Could you check a few things on this model? Use its own coordinates, in mm. Face numbers are marked on the shaded views. Round coordinates to 2 decimals unless told otherwise and drop trailing zeros. Write each question's results on one line, items separated by ' | '. Start each with the question number.
1) If I drill on probe 1 along X at (y, z) = (-11.8, 6.5); probe 2 along Z at (x, y) = (41.25, -11.3); probe 3 along Z at (x, y) = (42.75, -13.25), over which ranges is the centre line in solid material (lowest first)?
2) For P1, Ø3, axis at x = 44.5, z = 8, coming from the +Y side; P2, Ø1.5, axis at x = 44.5, z = 6, coming from the +Y side; P3, Ø1, axis at y = -11.5, z = 5.5, coming from the -X side, each with a flat end and sliding along its axis, tell me the tip position at first contact or that it passes through.
3) We'd pull the mould along Z, two halves only. Please class the marked faces 1 and 2: pulls with the +Z half, pulls with the -Z half, needs draft (parallel to the pull), parting line crosses it, or undercut.
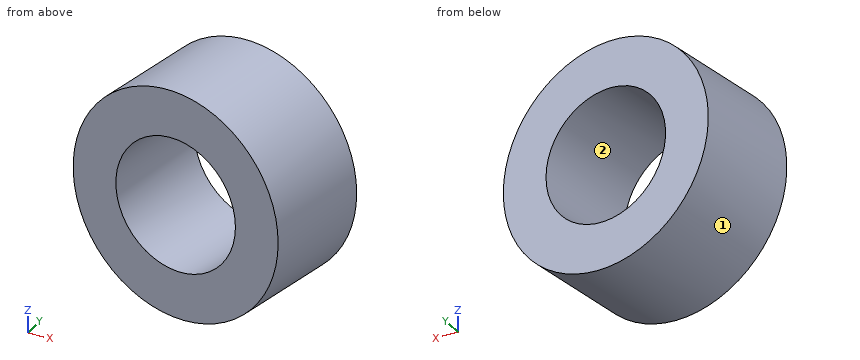
from build123d import *

# Parameters (mm, degrees)
CYLINDER044_R               = 1.75
CYLINDER044_DEPTH           = 18
CYLINDER044_ROLL_ANGLE      = -89.999776
CYLINDER044_PITCH_ANGLE     = 1.4e-05
CYLINDER044_PLACEMENT_ANGLE = -9.999925
CYLINDER045_R               = 3
CYLINDER045_DEPTH           = 3
CYLINDER045_ROLL_ANGLE      = -89.999776
CYLINDER045_PITCH_ANGLE     = 1.4e-05
CYLINDER045_PLACEMENT_ANGLE = -9.999925


with BuildPart() as cylinder044:
    # Cylinder044 → Cylinder044 (new body)
    with BuildSketch(Plane.XY):
        Circle(CYLINDER044_R)
    extrude(amount=CYLINDER044_DEPTH)


with BuildPart() as cylinder044_1:
    # Cylinder044 roll: moved
    add(cylinder044.part.rotate(Axis((0, 0, 0), (1, 0, 0)), CYLINDER044_ROLL_ANGLE))


with BuildPart() as cylinder044_2:
    # Cylinder044 pitch: moved
    add(cylinder044_1.part.rotate(Axis((0, 0, 0), (0, 1, 0)), CYLINDER044_PITCH_ANGLE))


with BuildPart() as cylinder044_3:
    # Cylinder044 placement: moved
    add(cylinder044_2.part.moved(Location((39.936529, -25.15494, 7.500007))).rotate(Axis((39.936529, -25.15494, 7.500007), (0, 0, 1)), CYLINDER044_PLACEMENT_ANGLE))


with BuildPart() as cut037:
    # Cylinder045 → Cylinder045 (new body)
    with BuildSketch(Plane.XY):
        Circle(CYLINDER045_R)
    extrude(amount=CYLINDER045_DEPTH)


with BuildPart() as cut037_1:
    # Cylinder045 roll: moved
    add(cut037.part.rotate(Axis((0, 0, 0), (1, 0, 0)), CYLINDER045_ROLL_ANGLE))


with BuildPart() as cut037_2:
    # Cylinder045 pitch: moved
    add(cut037_1.part.rotate(Axis((0, 0, 0), (0, 1, 0)), CYLINDER045_PITCH_ANGLE))


with BuildPart() as cut037_3:
    # Cylinder045 placement: moved
    add(cut037_2.part.moved(Location((42.020292, -13.337245, 7.500054))).rotate(Axis((42.020292, -13.337245, 7.500054), (0, 0, 1)), CYLINDER045_PLACEMENT_ANGLE))

    # Cut037: cut Cylinder044
    add(cylinder044_3.part, mode=Mode.SUBTRACT)


solid = cut037_3.part
Checked values:
1) probe 1: 39.42 to 40.83, 43.75 to 45.16 | probe 2: 4.71 to 6.15, 8.85 to 10.29 | probe 3: 4.58 to 5.9, 9.1 to 10.42
2) P1: y = -10.53 | P2: y = -10.6 | P3: x = 39.69
3) face 1: parting line crosses it | face 2: undercut
